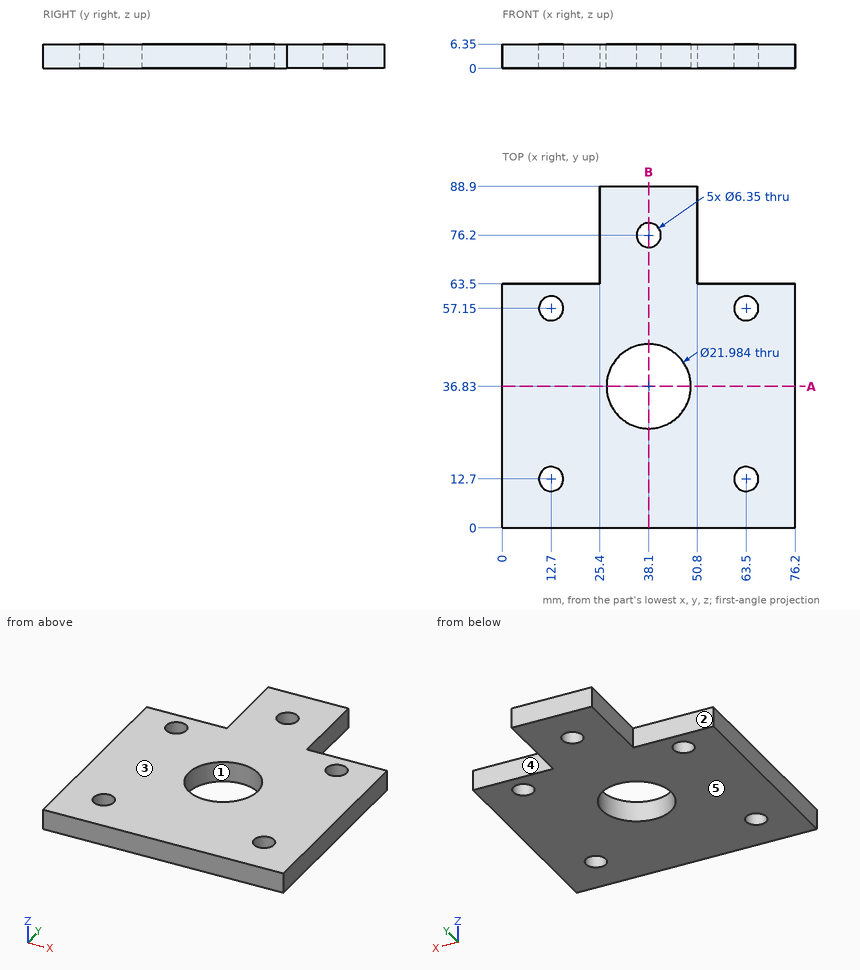
Check sheet for the drawn part. Datum: minimum x, y, z corner. Units: mm. A direction names the side the tool comes from. Round coordinates to 2 decimals unless told otherwise and drop trailing zeros. Loops run counter-clockwise (first coordinate to the right, second up) from the corner with the lowest first, then second, coordinate; pieces in that order, holes last. Notation, with made-up numbers: (6.5, 4.5) - (50.5, 4.5) arc R32 ccw to (50.5, 35.5) - close; hole circle Ø10 at (-33.5, -10.75). An arc over 180 degrees is marked (long way). Answer as a JSON object with one key per item and string values. Group by question number.
Q1. Mould release check, pull along Y, two halves, no side actions. Record for the marked faces 1, 2 and 3: released by +Y, released by -Y, zero draft, split by the parting line, or undercut.
Q2. Gauge pin test, flat ends, axial feed: P1, Ø1.9, axis at y = 74, z = 4, coming from the -X side; P2, Ø3, axis at x = 68, z = 4.5, coming from the +Y side. Record the tip position at first contact, or that the pin passes through.
Q3. Set-up check for the marked faces 4 and 5: record each of +Z, -Z, +X, -X, +Y, -Y from which the full face is reachable in a straight line by a thin tool's end or side.
Q4. Sectioned sample at B-B, the plane x = 38.1. Count the separate pieces of the cut face and the enclosed holes in it.
Q5. Scan lines: line 1 along Y through (x, z) = (38.1, 4.5) (1 decimal); line 2 along Y through (x, z) = (63.5, 2.5) (1 decimal); line 3 along X through (y, z) = (55, 5) (1 decimal). Record each from-to range of solid material in increasing order. Write a range as [from, to].
Q6. Sectioned sample at A-A, the plane y = 36.83. Enter the section's corners in (x, z), plus the area to 3 significant figures.
Solution:
{
 "1": {"face 1": "undercut", "face 2": "released by +Y", "face 3": "zero draft"},
 "2": {"P1": "stops at x = 25.4", "P2": "stops at y = 63.5"},
 "3": {"face 4": "+Z, -Z, +X, +Y", "face 5": "-Z, +X, -X, +Y, -Y"},
 "4": {"separate pieces": "3", "enclosed holes": "0"},
 "5": {"line 1": "y = [0, 25.8], [47.8, 73], [79.4, 88.9]", "line 2": "y = [0, 9.5], [15.9, 54], [60.3, 63.5]", "line 3": "x = [0, 10.4], [15, 61.2], [65.8, 76.2]"},
 "6": {"outline": "(0, 0) - (27.11, 0) - (27.11, 6.35) - (0, 6.35) - close; (49.09, 0) - (76.2, 0) - (76.2, 6.35) - (49.09, 6.35) - close", "area": "344 mm²"}
}
